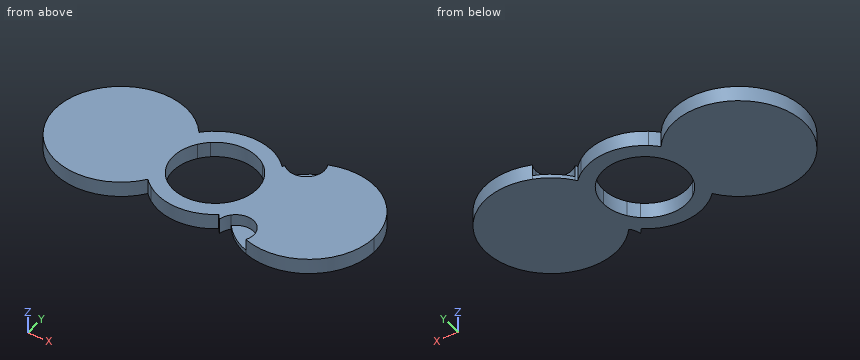
from build123d import *

# Parameters (mm, degrees)
F1_DEPTH = 4
F2_DEPTH = 1


# Not quite as in the source:
# - a feature names something its author has since deleted; it is built from what else it names


with BuildPart() as f1:
    # F0 (on Top) → F1 (new body)
    with BuildSketch(Plane.XY):
        with BuildLine():
            ThreePointArc((33.96875, 44.5973311111), (35.4798914594, 41.5709736662), (36, 38.228538177))
            ThreePointArc((36, 38.228538177), (35.4798914594, 34.8861026877), (33.96875, 31.8597452428))
            ThreePointArc((33.96875, 31.8597452428), (34.890304672, 29.9063024739), (36.04875, 28.083336186))
            ThreePointArc((36.04875, 28.083336186), (38.9773253879, 32.7847917648), (40, 38.228538177))
            ThreePointArc((40, 38.228538177), (38.9773253879, 43.6722845891), (36.04875, 48.3737401679))
            ThreePointArc((36.04875, 48.3737401679), (34.890304672, 46.55077388), (33.96875, 44.5973311111))
        make_face()
        with BuildLine():
            ThreePointArc((31.92, 46.7791872751), (33.0189287452, 45.7582647177), (33.96875, 44.5973311111))
            ThreePointArc((33.96875, 44.5973311111), (34.890304672, 46.55077388), (36.04875, 48.3737401679))
            ThreePointArc((36.04875, 48.3737401679), (35.0671824784, 49.3484229311), (34, 50.228538177))
            ThreePointArc((34, 50.228538177), (32.8729423014, 48.5563595633), (31.92, 46.7791872751))
        make_face()
        with BuildLine():
            ThreePointArc((36.04875, 28.083336186), (34.890304672, 29.9063024739), (33.96875, 31.8597452428))
            ThreePointArc((33.96875, 31.8597452428), (33.0189287452, 30.6988116362), (31.92, 29.6778890788))
            ThreePointArc((31.92, 29.6778890788), (32.8729423014, 27.9007167906), (34, 26.228538177))
            ThreePointArc((34, 26.228538177), (35.0671824784, 27.1086534228), (36.04875, 28.083336186))
        make_face()
        with BuildLine():
            ThreePointArc((18.08, 46.7791872751), (25, 49.228538177), (31.92, 46.7791872751))
            ThreePointArc((31.92, 46.7791872751), (32.8729423014, 48.5563595633), (34, 50.228538177))
            ThreePointArc((34, 50.228538177), (25, 53.228538177), (16, 50.228538177))
            ThreePointArc((16, 50.228538177), (17.1270576986, 48.5563595633), (18.08, 46.7791872751))
        make_face()
        with BuildLine():
            ThreePointArc((36.4851682331, 48.9482313775), (36.2639553749, 48.6632675964), (36.04875, 48.3737401679))
            ThreePointArc((36.04875, 48.3737401679), (38.9773253879, 43.6722845891), (40, 38.228538177))
            ThreePointArc((40, 38.228538177), (38.9773253879, 32.7847917648), (36.04875, 28.083336186))
            ThreePointArc((36.04875, 28.083336186), (36.2190453875, 27.853192883), (36.3931368718, 27.6259075689))
            ThreePointArc((36.3931368718, 27.6259075689), (41.5858805009, 28.7167510128), (44.5495147975, 24.3154560246))
            ThreePointArc((44.5495147975, 24.3154560246), (44.4052654508, 23.1537499865), (43.9812786211, 22.062601985))
            ThreePointArc((43.9812786211, 22.062601985), (59.8422445665, 24.0619323063), (67.25, 38.228538177))
            ThreePointArc((67.25, 38.228538177), (59.9032981891, 52.3525314146), (44.1210510171, 54.4458270643))
            ThreePointArc((44.1210510171, 54.4458270643), (44.5307176941, 53.3709710002), (44.6699958357, 52.2291549274))
            ThreePointArc((44.6699958357, 52.2291549274), (41.6873482182, 47.8201907003), (36.4851682331, 48.9482313775))
        make_face()
        with BuildLine():
            ThreePointArc((50, 45.978538177), (55.4800775542, 43.7086157311), (57.75, 38.228538177))
            ThreePointArc((57.75, 38.228538177), (44.5199224458, 32.7484606228), (50, 45.978538177))
        make_face(mode=Mode.SUBTRACT)
        with BuildLine():
            ThreePointArc((34, 26.228538177), (32.8729423014, 27.9007167906), (31.92, 29.6778890788))
            ThreePointArc((31.92, 29.6778890788), (25, 27.228538177), (18.08, 29.6778890788))
            ThreePointArc((18.08, 29.6778890788), (17.1270576986, 27.9007167906), (16, 26.228538177))
            ThreePointArc((16, 26.228538177), (25, 23.228538177), (34, 26.228538177))
        make_face()
        with BuildLine():
            ThreePointArc((36.3931368718, 27.6259075689), (36.2190453875, 27.853192883), (36.04875, 28.083336186))
            ThreePointArc((36.04875, 28.083336186), (35.0671824784, 27.1086534228), (34, 26.228538177))
            ThreePointArc((34, 26.228538177), (34.528786958, 25.5540927449), (35.0859826327, 24.9029205189))
            ThreePointArc((35.0859826327, 24.9029205189), (35.517354176, 26.3710825501), (36.3931368718, 27.6259075689))
        make_face()
        with BuildLine():
            ThreePointArc((16.03125, 44.5973311111), (16.9810712548, 45.7582647177), (18.08, 46.7791872751))
            ThreePointArc((18.08, 46.7791872751), (17.1270576986, 48.5563595633), (16, 50.228538177))
            ThreePointArc((16, 50.228538177), (14.9328175216, 49.3484229311), (13.95125, 48.3737401679))
            ThreePointArc((13.95125, 48.3737401679), (15.109695328, 46.55077388), (16.03125, 44.5973311111))
        make_face()
        with BuildLine():
            ThreePointArc((16, 26.228538177), (17.1270576986, 27.9007167906), (18.08, 29.6778890788))
            ThreePointArc((18.08, 29.6778890788), (16.9810712548, 30.6988116362), (16.03125, 31.8597452428))
            ThreePointArc((16.03125, 31.8597452428), (15.109695328, 29.9063024739), (13.95125, 28.083336186))
            ThreePointArc((13.95125, 28.083336186), (14.9328175216, 27.1086534228), (16, 26.228538177))
        make_face()
        with BuildLine():
            ThreePointArc((16.03125, 31.8597452428), (14, 38.228538177), (16.03125, 44.5973311111))
            ThreePointArc((16.03125, 44.5973311111), (15.109695328, 46.55077388), (13.95125, 48.3737401679))
            ThreePointArc((13.95125, 48.3737401679), (10, 38.228538177), (13.95125, 28.083336186))
            ThreePointArc((13.95125, 28.083336186), (15.109695328, 29.9063024739), (16.03125, 31.8597452428))
        make_face()
        with BuildLine():
            ThreePointArc((13.95125, 28.083336186), (10, 38.228538177), (13.95125, 48.3737401679))
            ThreePointArc((13.95125, 48.3737401679), (-17.25, 38.228538177), (13.95125, 28.083336186))
        make_face()
        with BuildLine():
            ThreePointArc((0, 45.978538177), (5.4800775542, 43.7086157311), (7.75, 38.228538177))
            ThreePointArc((7.75, 38.228538177), (-5.4800775542, 32.7484606228), (0, 45.978538177))
        make_face(mode=Mode.SUBTRACT)
        with BuildLine():
            ThreePointArc((0, 45.978538177), (-5.4800775542, 32.7484606228), (7.75, 38.228538177))
            ThreePointArc((7.75, 38.228538177), (5.4800775542, 43.7086157311), (0, 45.978538177))
        make_face()
        with BuildLine():
            ThreePointArc((50, 45.978538177), (44.5199224458, 32.7484606228), (57.75, 38.228538177))
            ThreePointArc((57.75, 38.228538177), (55.4800775542, 43.7086157311), (50, 45.978538177))
        make_face()
    extrude(amount=F1_DEPTH)

    # F0 (on Top) → F2 (join)
    with BuildSketch(Plane.XY):
        with BuildLine():
            ThreePointArc((44.1210510171, 54.4458270643), (39.9210331617, 52.2277141339), (36.4851682331, 48.9482313775))
            ThreePointArc((36.4851682331, 48.9482313775), (41.6873482182, 47.8201907003), (44.6699958357, 52.2291549274))
            ThreePointArc((44.6699958357, 52.2291549274), (44.5307176941, 53.3709710002), (44.1210510171, 54.4458270643))
        make_face()
        with BuildLine():
            ThreePointArc((44.5495147975, 24.3154560246), (41.5858805009, 28.7167510128), (36.3931368718, 27.6259075689))
            ThreePointArc((36.3931368718, 27.6259075689), (39.8005645222, 24.31688781), (43.9812786211, 22.062601985))
            ThreePointArc((43.9812786211, 22.062601985), (44.4052654508, 23.1537499865), (44.5495147975, 24.3154560246))
        make_face()
    extrude(amount=F2_DEPTH)


solid = f1.part
Build history of the part. All positions in model axes, mm. Give positions to 0.01 mm unless a question says otherwise; leave off trailing zeros. Write each loop counter-clockwise with the first axis right and the second up, starting at its lowest first coordinate (ties: lowest second). Pieces come first, ordered by that corner, then holes. Notation, with made-up numbers: (62.25, 83.25) - (71.25, 83.25) arc R19 cw to (71.25, 104.25) - close; hole circle Ø2 at (52, 41). An arc over 180 degrees is marked (long way). Use one line per item in the form item = value. Start each with the question number.
1. Probe line 1 (Y direction, x = 25, z = 1.55); line 2 (X direction, y = 50, z = 1.85); line 3 (X direction, y = 28.5, z = 3.05). List the from-to ranges inside material, lowest first. Write a range as [from, to].
2. Band-saw the part on D-D on x = 12. Write the cut outline in (y, z).
3. Band-saw the part on A-A on z = 2.15. Write the cut outline in (x, y), plus the area to 3 significant figures.
4. Drop flat-ended pins along their axis: pin 1 Ø12 at (x, y) = (-4.5, 48) entering from -Z; pin 2 Ø1.5 at (x, z) = (44, 2) entering from +Y; pin 3 Ø3.5 at (x, y) = (41, 49.5) entering from +Z. Give the stop position or say it passes through.
5. Band-saw the part on B-B on x = 33. Write the cut outline in (y, z).
6. Band-saw the part on C-C on y = 31. Write the cut outline in (x, z), plus the area to 3 significant figures.
Conclusion:
q1.line_1 = [23.23, 27.23], [49.23, 53.23]
q1.line_2 = [-12.61, 12.61], [15.7, 34.3], [44.11, 62.61]
q1.line_3 = [-14.24, 19.87], [30.13, 37.55], [42.05, 64.24]
q2.outline = (25.84, 0) - (50.62, 0) - (50.62, 4) - (25.84, 4) - close
q3.outline = (13.95, 28.08) arc R15 ccw to (34, 26.23) arc R20 ccw to (35.09, 24.9) arc R4.75 cw (long way) to (43.98, 22.06) arc R17.25 ccw (long way) to (44.12, 54.45) arc R4.75 cw to (36.49, 48.95) arc R17.25 ccw to (36.05, 48.37) arc R15 ccw to (13.95, 48.37) arc R17.25 ccw (long way) to start; hole circle Ø22 at (25, 38.23)
q3.area = 1,930 mm²
q4.pin_1 = 0
q4.pin_2 = 54.66
q4.pin_3 = 1
q5.outline = (25.54, 0) - (30.68, 0) - (30.68, 4) - (25.54, 4) - close; (45.78, 0) - (50.92, 0) - (50.92, 4) - (45.78, 4) - close
q6.outline = (-15.66, 0) - (16.71, 0) - (16.71, 4) - (-15.66, 4) - close; (33.29, 0) - (65.66, 0) - (65.66, 4) - (33.29, 4) - close
q6.area = 259 mm²
